Could you check a few things on this model? Use its own coordinates, in mm. A direction names the side the tool comes from. Give positions to 0.01 mm unless a question says otherwise; leave off trailing zeros. Order: outer loops, then holes, each group sorted by start corner. A loop starts at its lowest first (then second) coordinate and runs counter-clockwise, first axis right, second up. Notation, with made-up numbers: (9.5, -35) - (64.5, -35) arc R19 ccw to (64.5, -19) - close; hole circle Ø9 at (44, -21). An arc over 180 degrees is marked (long way). Put each result on its own line as item: value.
from build123d import *

# Parameters (mm, degrees)
BOX018_W               = 16
BOX018_H               = 4
BOX018_DEPTH           = 43
BOX018_PLACEMENT_ANGLE = 18
BOX017_W               = 16
BOX017_H               = 4
BOX017_DEPTH           = 43
BOX017_PLACEMENT_ANGLE = 18
BOX014_W               = 11
BOX014_H               = 4
BOX014_DEPTH           = 34
BOX015_W               = 11
BOX015_H               = 4
BOX015_DEPTH           = 34
BOX016_W               = 13
BOX016_H               = 4
BOX016_DEPTH           = 10
BOX013_W               = 35
BOX013_H               = 4
BOX013_DEPTH           = 14


with BuildPart() as obj1:
    # Box018 → Box018 (new body)
    with BuildSketch(Plane.XY):
        with Locations((8, 2)):
            Rectangle(BOX018_W, BOX018_H)
    extrude(amount=BOX018_DEPTH)


with BuildPart() as obj1_1:
    # Box018 placement: moved
    add(obj1.part.moved(Location((39, 0, 9))).rotate(Axis((39, 0, 9), (0, -1, 0)), BOX018_PLACEMENT_ANGLE))


with BuildPart() as fusion010:
    # Box017 → Box017 (new body)
    with BuildSketch(Plane.XY):
        with Locations((8, 2)):
            Rectangle(BOX017_W, BOX017_H)
    extrude(amount=BOX017_DEPTH)


with BuildPart() as fusion010_1:
    # Box017 placement: moved
    add(fusion010.part.moved(Location((-15, 0, 14))).rotate(Axis((-15, 0, 14), (0, 1, 0)), BOX017_PLACEMENT_ANGLE))

    # Fusion010: union obj1
    add(obj1_1.part)


with BuildPart() as obj2:
    # Box014 → Box014 (new body)
    with BuildSketch(Plane(origin=(2, 0, 14), x_dir=(1, 0, 0), z_dir=(0, 0, 1))):
        with Locations((5.5, 2)):
            Rectangle(BOX014_W, BOX014_H)
    extrude(amount=BOX014_DEPTH)


with BuildPart() as obj3:
    # Box015 → Box015 (new body)
    with BuildSketch(Plane(origin=(26, 0, 14), x_dir=(1, 0, 0), z_dir=(0, 0, 1))):
        with Locations((5.5, 2)):
            Rectangle(BOX015_W, BOX015_H)
    extrude(amount=BOX015_DEPTH)


with BuildPart() as obj4:
    # Box016 → Box016 (new body)
    with BuildSketch(Plane(origin=(13, 0, 38), x_dir=(1, 0, 0), z_dir=(0, 0, 1))):
        with Locations((6.5, 2)):
            Rectangle(BOX016_W, BOX016_H)
    extrude(amount=BOX016_DEPTH)


with BuildPart() as cut004:
    # Box013 → Box013 (new body)
    with BuildSketch(Plane(origin=(2, 0, 0), x_dir=(1, 0, 0), z_dir=(0, 0, 1))):
        with Locations((17.5, 2)):
            Rectangle(BOX013_W, BOX013_H)
    extrude(amount=BOX013_DEPTH)

    # Fusion009: union obj2, obj3, obj4
    add(obj2.part)
    add(obj3.part)
    add(obj4.part)

    # Cut004: cut Fusion010
    add(fusion010_1.part, mode=Mode.SUBTRACT)


with BuildPart() as cut004_1:
    # Cut004 placement: moved
    add(cut004.part.moved(Location((21, 23, -7))))


solid = cut004_1.part
1) Suppose I cut it at D-D, the plane x = 27. List the corners of the cut face in (y, z) for me.
Filled in:
outline: (23, -7) - (27, -7) - (27, 19.85) - (23, 19.85) - close
2) Suppose I cut it at B-B, the plane z = 25.5. List the corners of the cut face in (x, y) for me, and give its area (3 significant figures).
Filled in:
outline: (28.83, 23) - (34, 23) - (34, 27) - (28.83, 27) - close; (47, 23) - (52.36, 23) - (52.36, 27) - (47, 27) - close
area: 42.1 mm^2
3) I'm going to push flat-ended pins straight in: pin 1 (2 mm diameter, centred on y = 25, z = 18.5, fed in from -X); pin 2 (1 mm diameter, centred on y = 25, z = 28.5, fed in from -X); pin 3 (2 mm diameter, centred on y = 24.5, z = 21.5, fed in from +X). Where does each tip first touch, or does it pass through?
Filled in:
pin 1: stops at x = 26.24
pin 2: stops at x = 29.65
pin 3: stops at x = 53.99
4) We'd pull the mould along X, two halves only. Please class faces 1 (the flat face through (28.36, 24.97, 24.04)), 2 (the flat face through (40, 25, 31)), 3 (the flat face through (52.74, 24.97, 24.35)): pulls with the +X half, pulls with the -X half, needs draft (parallel to the pull), parting line crosses it, or undercut.
Filled in:
face 1: pulls with the -X half
face 2: undercut
face 3: pulls with the +X half
5) Which directions (+Z, -Z, +X, -X, +Y, -Y) give clear straight access to the entire face, cutting with the end or side of a thin tool? Please do faces 4 (the flat face through (58, 25, 0)), 5 (the flat face through (34, 25, 19)).
Filled in:
face 4: +Z, -Z, +X, +Y, -Y
face 5: +Y, -Y
6) Suppose I cut it at A-A, the plane x = 43.5. List the corners of the cut face in (y, z) for me.
Filled in:
outline: (23, -7) - (27, -7) - (27, 7) - (23, 7) - close; (23, 31) - (27, 31) - (27, 41) - (23, 41) - close
7) Suppose I cut it at C-C, the plane y = 25.2. List the corners of the cut face in (x, z) for me.
Filled in:
outline: (23, -7) - (58, -7) - (58, 8.16) - (47.33, 41) - (33.87, 41) - (23, 7.54) - close; hole (34, 7) - (47, 7) - (47, 31) - (34, 31) - close
8) If I drill on line 1 (Z direction, x = 37, y = 23.3); line 2 (X direction, y = 26.1, z = 27); line 3 (X direction, y = 25.95, z = 19), over which ranges is the centre line in solid material (lowest first)? Write a range as [from, to].
Filled in:
line 1: z = [-7, 7], [31, 41]
line 2: x = [29.32, 34], [47, 51.88]
line 3: x = [26.72, 34], [47, 54.48]
